Check sheet for the modelled part. Datum: model origin and axes. Units: mm. Give positions to 0.01 mm unless a question says otherwise; leave off trailing zeros. Loops run counter-clockwise (first coordinate to the right, second up) from the corner with the lowest first, then second, coordinate; pieces in that order, holes last. Notation, with made-up numbers: (54.5, 30.25) -> (105.5, 30.25) arc R20 ccw to (105.5, 66.25) -> close; hole circle Ø10 at (73, -25.75). An arc over 180 degrees is marked (long way). Write each question's results on one line, items separated by ' | '. Start each with the question number.
1. Cross-section at B-B on z = 5. Record the boundary of the cut face in (x, y), and give its area (3 significant figures).
2. Mould release check, pull along Z, two halves, no side actions. Record for faces 1 (the face through (-5, -1.5, 5)), 2 (the face through (0, 0, 0)), 3 (the face through (-15, 0, 5)), 4 (the face through (0.09, -0.02, 2.95)): +Z half, -Z half, draft (parallel to the pull), parting line (faces both ways), or undercut.
3. Cross-section at C-C on y = -2.75. Record the boundary of the cut face in (x, z).
4. Gauge pin test, flat ends, axial feed: pin 1 Ø1 at (y, z) = (-1, 8) entering from +X; pin 2 Ø3.5 at (x, z) = (-10, 5) entering from -Y; pin 3 Ø3 at (y, z) = (0, 3) entering from -X; pin 4 Ø5 at (y, z) = (0, 1) entering from -X. Record the tip position at first contact, or that the pin passes through.
5. Material ranges on L1, parallel to X at y = 0.3, z = 5; L2, parallel to X at y = -1, z = 4; L3, parallel to Y at x = -13, z = 8, recorded low to high. Write a range as from..to.
6. Cross-section at A-A on x = 0. Record the boundary of the cut face in (y, z), and give its area (3 significant figures).
7. Cross-section at D-D on x = -3.75. Record the boundary of the cut face in (y, z).
from build123d import *
from build123d.topology import SkipClean

# Parameters (mm, degrees)
SKETCH1_R           = 2.05
BOSS_EXTRUDE1_DEPTH = 1.5
SKETCH2_R           = 5
SKETCH2_R_2         = 2.05
BOSS_EXTRUDE2_DEPTH = 3


with BuildPart() as part:
    # Sketch1 → Boss-Extrude1 (new, symmetric)
    with BuildSketch(Plane(origin=(0, 0, 0), x_dir=(1, 0, 0), z_dir=(0, 1, 0))):
        with BuildLine():
            Line((-10, 0), (-5, 0))
            Line((-5, 0), (5, 0))
            Line((5, 0), (10, 0))
            ThreePointArc((10, 0), (15, -5), (10, -10))
            Line((10, -10), (5, -10))
            Line((5, -10), (-5, -10))
            Line((-5, -10), (-10, -10))
            ThreePointArc((-10, -10), (-15, -5), (-10, 0))
        make_face()
        with Locations(Location((10, -5, 0), (0, 0, 270))):
            Circle(SKETCH1_R, mode=Mode.SUBTRACT)
        with Locations(Location((-10, -5, 0), (0, 0, 90))):
            Circle(SKETCH1_R, mode=Mode.SUBTRACT)
        with Locations(Location((0, -5, 0), (0, 0, 270))):
            Circle(SKETCH1_R, mode=Mode.SUBTRACT)
    extrude(amount=BOSS_EXTRUDE1_DEPTH, both=True)

    # Sketch2 → Boss-Extrude2 (add)
    with BuildSketch(Plane(origin=(0, 1.5, 0), x_dir=(1, 0, 0), z_dir=(0, 1, 0))):
        with Locations(Location((10, -5, 0), (0, 0, 270))):
            Circle(SKETCH2_R)
        with Locations(Location((10, -5, 0), (0, 0, 270))):
            Circle(SKETCH2_R_2, mode=Mode.SUBTRACT)
    boss_extrude2 = extrude(amount=BOSS_EXTRUDE2_DEPTH)

    # Mirror1: Boss-Extrude2 across plane
    with SkipClean():  # the faces are left unmerged after this step: merging them gives an invalid solid
        add(boss_extrude2.mirror(Plane.ZX))


solid = part.part
Geometry says:
1) outline: (-15, -1.5) -> (-12.05, -1.5) -> (-12.05, 1.5) -> (-15, 1.5) -> close; (-7.95, -1.5) -> (-2.05, -1.5) -> (-2.05, 1.5) -> (-7.95, 1.5) -> close; (2.05, -1.5) -> (5, -1.5) -> (5, -4.5) -> (7.95, -4.5) -> (7.95, 4.5) -> (5, 4.5) -> (5, 1.5) -> (2.05, 1.5) -> close; (12.05, -4.5) -> (15, -4.5) -> (15, 4.5) -> (12.05, 4.5) -> close | area: 88.5 mm^2
2) face 1: draft | face 2: -Z half | face 3: parting line | face 4: undercut
3) outline: circle Ø10 at (10, 5); hole circle Ø4.1 at (10, 5)
4) pin 1: x = 14.33 | pin 2: through | pin 3: x = -14.97 | pin 4: x = -14.77
5) L1: -15..-12.05, -7.95..-2.05, 2.05..7.95, 12.05..15 | L2: -14.9..-11.79, -8.21..-1.79, 1.79..8.21, 11.79..14.9 | L3: -1.5..1.5
6) outline: (-1.5, 0) -> (1.5, 0) -> (1.5, 2.95) -> (-1.5, 2.95) -> close; (-1.5, 7.05) -> (1.5, 7.05) -> (1.5, 10) -> (-1.5, 10) -> close | area: 17.7 mm^2
7) outline: (-1.5, 0) -> (1.5, 0) -> (1.5, 10) -> (-1.5, 10) -> close
